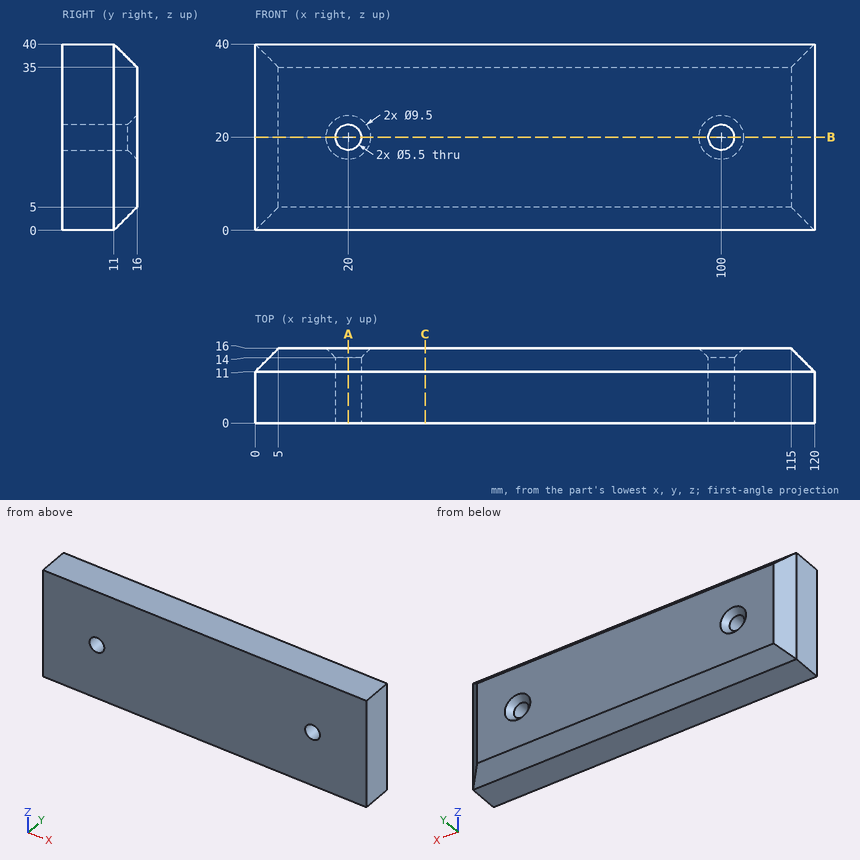
Could you check a few things on this drawing? It's one solid part, dimensions in mm from its lowest x, y, z. Give positions to 0.01 mm unless a question says otherwise; leave off trailing zeros. Order: outer loops, then holes, each group sorted by start corner. A loop starts at its lowest first (then second) coordinate and runs counter-clockwise, first axis right, second up. Notation, with made-up numbers: (-21.5, 31) - (-14.5, 31) arc R13 cw to (-14.5, 42) - close; hole circle Ø9 at (75, -8). An arc over 180 degrees is marked (long way). Return JSON: item names as keys, results as strings. Group by question number.
Q1. Will these pins go through, and if not, where does the flat tip stop? pin 1 Ø12 at (x, z) = (36.5, 20.5) entering from -Y; pin 2 Ø1 at (y, z) = (13, 5) entering from -X.
Q2. Suppose I cut it at B-B, the plane z = 20. Please give me the cut outline in (x, y).
Q3. Suppose I cut it at C-C, the plane x = 36.5. Please give me the cut outline in (y, z), and give its area (3 significant figures).
Q4. Suppose I cut it at A-A, the plane x = 20. Please give me the cut outline in (y, z), and give its area (3 significant figures).
Q5. Please list where these lines run through material, in increasing order: line 1 along X through (y, z) = (6.25, 20); line 2 along Z through (x, y) = (20, 10.25); line 3 along X through (y, z) = (12.5, 20). Write a range as [from, to].
Resolved:
{
 "1": {"pin 1": "stops at y = 0", "pin 2": "stops at x = 1.5"},
 "2": {"outline": "(0, 0) - (17.25, 0) - (17.25, 14) - (15.25, 16) - (5, 16) - (0, 11) - close; (22.75, 0) - (97.25, 0) - (97.25, 14) - (95.25, 16) - (24.75, 16) - (22.75, 14) - close; (102.75, 0) - (120, 0) - (120, 11) - (115, 16) - (104.75, 16) - (102.75, 14) - close"},
 "3": {"outline": "(0, 0) - (11, 0) - (16, 5) - (16, 35) - (11, 40) - (0, 40) - close", "area": "615 mm2"},
 "4": {"outline": "(0, 0) - (11, 0) - (16, 5) - (16, 15.25) - (14, 17.25) - (0, 17.25) - close; (0, 22.75) - (14, 22.75) - (16, 24.75) - (16, 35) - (11, 40) - (0, 40) - close", "area": "523 mm2"},
 "5": {"line 1": "x = [0, 17.25], [22.75, 97.25], [102.75, 120]", "line 2": "z = [0, 17.25], [22.75, 40]", "line 3": "x = [1.5, 17.25], [22.75, 97.25], [102.75, 118.5]"}
}
